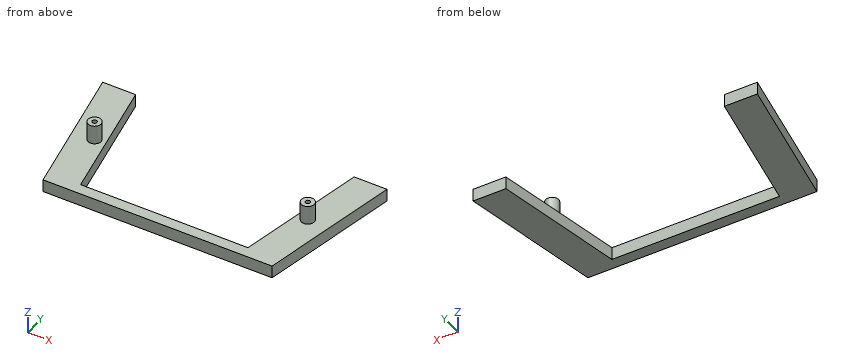
Autodesk Inventor part; units mm, degrees
ref_plane "YZ Plane" through (0, 0, 0) normal (1, 0, 0) x (0, 1, 0)
ref_plane "XZ Plane" through (0, 0, 0) normal (0, 1, 0) x (-1, 0, 0)
ref_plane "XY Plane" through (0, 0, 0) normal (0, 0, 1) x (1, 0, 0)
sketch "Sketch1" plane through (0, 0, 0) normal (0, 0, 1) x (1, 0, 0)
  line L0 (-36.2529, -22.5) -> (36.2529, -22.5)
  line L1 (36.2529, -22.5) -> (45, 22.5)
  line L2 (45, 22.5) -> (-45, 22.5)
  line L3 (-45, 22.5) -> (-36.2529, -22.5)
  point P0 (0, 0)
  point P1 (0, -22.5)
  point P2 (40.6264, 0)
  point P3 (0, 22.5)
  dimension "d0" = 45
  dimension "d1" = 22
  dimension "d2" = 90
extrude "Extrusion1" add sketch "Sketch1" along normal blind 4
sketch "Sketch2" plane through (0, 0, 4) normal (0, 0, 1) x (1, 0, 0)
  line L0 (-33.75, 0) -> (33.75, 0) construction
  circle A0 centre (33.75, 0) radius 2.05
  circle A1 centre (-33.75, 0) radius 2.05
  line L1 (45, 22.5) -> (-45, 22.5)
  line L2 (-36.2529, -22.5) -> (36.2529, -22.5)
  circle A2 centre (33.75, 0) radius 0.75
  circle A3 centre (-33.75, 0) radius 0.75
  point P0 (0, 0)
  point P1 (0, 0)
  dimension "d5" = 67.5
  dimension "d6" = 4.1
  dimension "d7" = 22.5
  dimension "d8" = 45
  dimension "d9" = 1.5
extrude "Extrusion2" add sketch "Sketch2" along normal blind 6
sketch "Sketch3" plane through (0, 0, 4) normal (0, 0, 1) x (1, 0, 0)
  line L0 (-26.5068, -19) -> (26.5068, -19)
  line L1 (26.5068, -19) -> (34.5736, 22.5)
  line L2 (34.5736, 22.5) -> (-34.5736, 22.5)
  line L3 (-34.5736, 22.5) -> (-26.5068, -19)
  line L4 (-45, 22.5) -> (-36.2529, -22.5)
  line L5 (36.2529, -22.5) -> (45, 22.5)
  line L6 (-30.2, 0) -> (30.2, 0) construction
  circle A0 centre (33.75, 0) radius 2.05
  line L7 (45, 22.5) -> (-45, 22.5)
  circle A1 centre (33.75, 0) radius 0.75
  point P0 (0, 0)
  point P1 (0, -19)
  dimension "d13" = 60.4
  dimension "d14" = 19
extrude "Extrusion3" cut sketch "Sketch3" against normal through all contours L3 L2 L1 L0
sketch "Sketch4" plane through (0, 0, 4) normal (0, 0, 1) x (1, 0, 0)
  line L0 (37.1379, 16.0576) -> (37.8822, 19.7792) construction
  line L1 (35.8639, 16.3124) -> (36.6083, 20.034)
  line L2 (39.1561, 19.5244) -> (38.4118, 15.8028)
  arc A0 (35.8639, 16.3124) -> (38.4118, 15.8028) centre (37.1379, 16.0576) ccw
  arc A1 (39.1561, 19.5244) -> (36.6083, 20.034) centre (37.8822, 19.7792) ccw
  point P0 (0, 0)
  point P1 (37.51, 17.9184)
equation "\"d7\" = 0.5 * d8"
properties part number "Touchpad Top"
Input: part model. Units: mm. Frame: model coordinates. Coordinates: 2 decimals unless noted, no trailing zeros. Loops run counter-clockwise (first coordinate to the right, second up) from the corner with the lowest first, then second, coordinate; pieces in that order, holes last.
Q1. Section B-B, the plane z = 7. Return the cut outline in (x, y).
Results are:
outline: circle Ø4.1 at (-33.75, 0); circle Ø4.1 at (33.75, 0); hole circle Ø1.5 at (-33.75, 0); hole circle Ø1.5 at (33.75, 0)
Q2. Contact query for flat-ended pins moving along their axis: pin 1 (3 mm diameter, centred on x = -33, z = 7.5, fed in from +Y); pin 2 (3 mm diameter, centred on x = 13, z = 2, fed in from +Y); pin 3 (8 mm diameter, centred on x = 33.5, y = 14.5, fed in from +Z). Output: stop coordinate, or through.
Results are:
pin 1: stops at y = 2.05
pin 2: stops at y = -19
pin 3: stops at z = 4
Q3. Line query: line 1 along Y through (x, z) = (33.75, 6.75); line 2 along Z through (x, y) = (-40, 10); line 3 along X through (y, z) = (-5, 2.25). Output: solid intervals per line, ascending.
Results are:
line 1: y = -2.05 to -0.75, 0.75 to 2.05
line 2: z = 0 to 4
line 3: x = -39.65 to -29.23, 29.23 to 39.65
Q4. Section C-C, the plane z = 3. Return the cut outline in (x, y).
Results are:
outline: (-45, 22.5) - (-36.25, -22.5) - (36.25, -22.5) - (45, 22.5) - (34.57, 22.5) - (26.51, -19) - (-26.51, -19) - (-34.57, 22.5) - close
Q5. Section D-D, the plane x = -11. Return the cut outline in (y, z), and give its area (3 significant figures).
Results are:
outline: (-22.5, 0) - (-19, 0) - (-19, 4) - (-22.5, 4) - close
area: 14.0 mm2
Q6. Section A-A, the plane y = -9.5. Return the cut outline in (x, z), and give its area (3 significant figures).
Results are:
outline: (-38.78, 0) - (-28.35, 0) - (-28.35, 4) - (-38.78, 4) - close; (28.35, 0) - (38.78, 0) - (38.78, 4) - (28.35, 4) - close
area: 83.4 mm2
